The drawing under review shows one solid part. Ordinate dimensions are in mm from its lowest x, y, z. Round coordinates to 2 decimals unless told otherwise and drop trailing zeros. Order: outer loops, then holes, each group sorted by start corner. A loop starts at its lowest first (then second) coordinate and runs counter-clockwise, first axis right, second up. Notation, with made-up numbers: M 15.5,18 L 29.5,18 A18 cw 29.5,44 Z; hole C 28.5,77.5 d7. An arc over 180 degrees is marked long. Use a Markdown table: item, result.
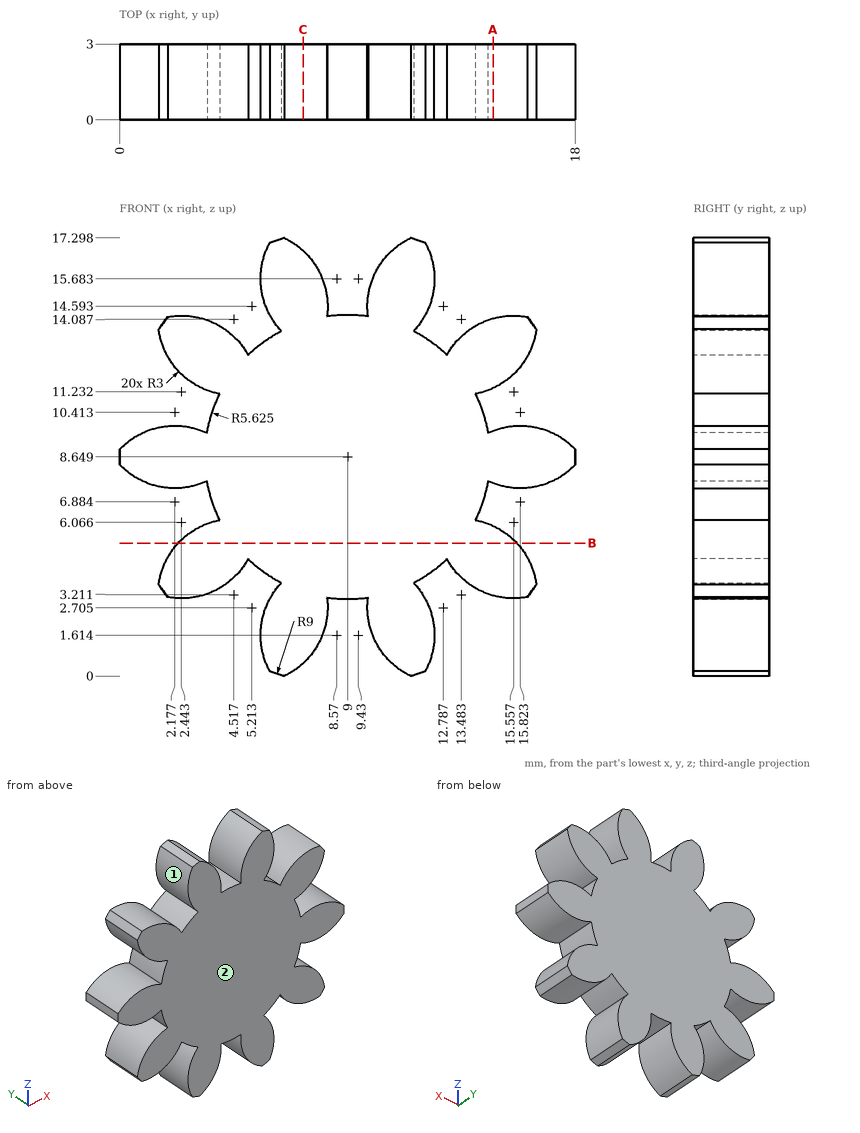
Q1. Draft analysis for pull direction Z (two halves, no side actions). For the marked faces 1 and 2, state which applies: pulls with the +Z half, pulls with the -Z half, needs draft (parallel to the pull), parting line crosses it, or undercut.
Determined:
| item | result |
|---|---|
| face 1 | undercut |
| face 2 | needs draft |
Q2. Add section A-A (x = 14.75). Write out the cut boundary in (y, z) (1 decimal).
Determined:
| item | result |
|---|---|
| outline | M 0,3.2 L 3,3.2 L 3,5.9 L 0,5.9 Z; M 0,7.6 L 3,7.6 L 3,9.7 L 0,9.7 Z; M 0,11.4 L 3,11.4 L 3,14.1 L 0,14.1 Z |
Q3. Add section C-C (x = 7.25). Write out the cut boundary in (y, z) (1 decimal).
Determined:
| item | result |
|---|---|
| outline | M 0,0.5 L 3,0.5 L 3,16.8 L 0,16.8 Z |
Q4. Add section B-B (z = 5.25). Write out the cut boundary in (x, y), then the cut area to 3 significant figures.
Determined:
| item | result |
|---|---|
| outline | M 2.32,0 L 15.68,0 L 15.68,3 L 2.32,3 Z |
| area | 40.1 mm^2 |
Q5. Wall thickness on line 1 along Z through (x, y) = (15.25, 0.75) (1 decimal); line 2 along X through (y, z) = (2.2, 4.5); line 3 along Z through (x, y) = (6, 0.35) (1 decimal): over which ranges is each line inside the solid? List them lowest first. Write a range as [from, to].
Determined:
| item | result |
|---|---|
| line 1 | z = [3.1, 5.6], [7.5, 9.8], [11.7, 14.2] |
| line 2 | x = [1.81, 5], [5.2, 12.8], [13, 16.19] |
| line 3 | z = [0.2, 3.2], [3.9, 13.4], [14.1, 17.1] |
